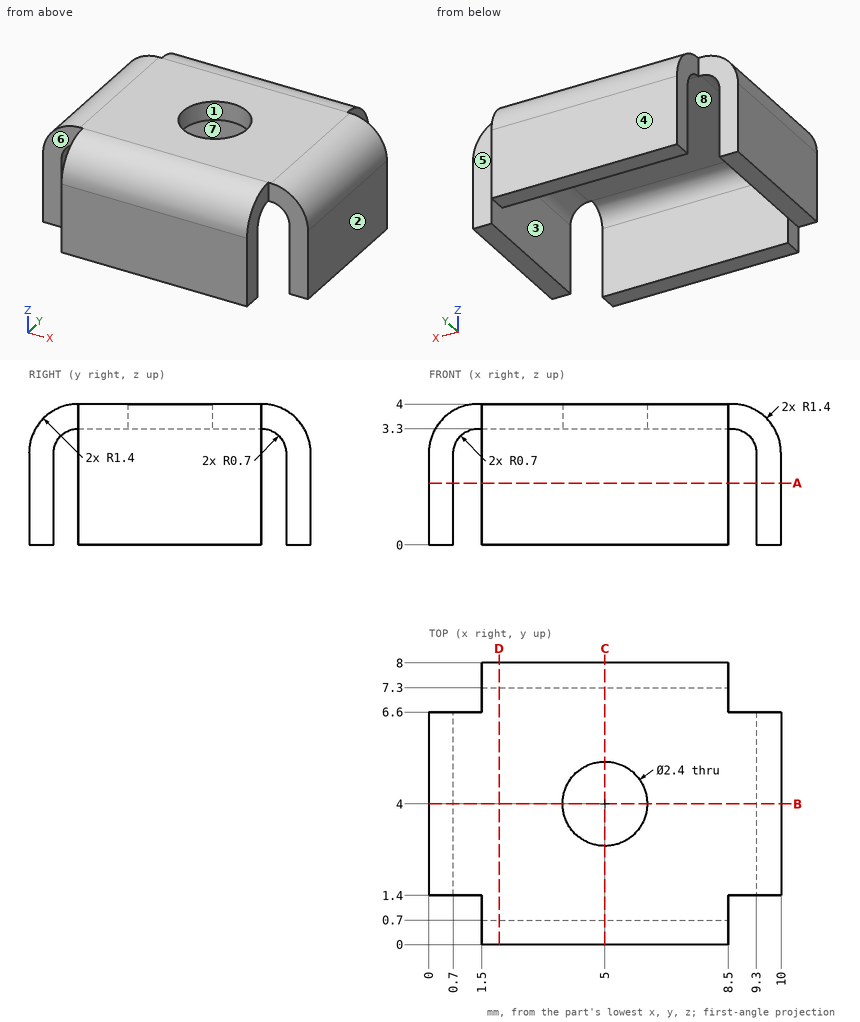
Geometry check sheet. Reference: drawing and pictorial views, mm from the part's lowest x, y, z. A direction names the side the tool comes from. Give positions to 0.01 mm unless a question says otherwise; leave off trailing zeros. Order: outer loops, then holes, each group sorted by start corner. A loop starts at its lowest first (then second) coordinate and runs counter-clockwise, first axis right, second up. Notation, with made-up numbers: (-2.5, 3) -> (2.5, 3) arc R25 cw to (2.5, 42) -> close; hole circle Ø11 at (87, 52). An arc over 180 degrees is marked (long way). Write each question's results on one line, items separated by ' | '. Start each with the question number.
(1) Mould release check, pull along X, two halves, no side actions. Record for the marked faces 1, 2, 3 and 4: pulls with the +X half, pulls with the -X half, needs draft (parallel to the pull), parting line crosses it, or undercut.
(2) Access from +Z, -Z, +X, -X, +Y, -Y to the whole of each face (thin tool, end or side, straight path). Record for the marked faces 5, 6, 7 and 8.
(3) Sectioned sample at A-A (z = 1.75). Enter the section's corners in (x, y).
(4) Gauge pin test, flat ends, axial feed: P1, Ø0.8, axis at x = 1, z = 2, coming from the -Y side; P2, Ø1.5, axis at y = 0.5, z = 2.5, coming from the -X side; P3, Ø0.5, axis at x = 0.5, z = 2, coming from the +Y side. Record the tip position at first contact, or that the pin passes through.
(5) Sectioned sample at C-C (x = 5). Enter the section's corners in (y, z), plus the area to 3 significant figures.
(6) Sectioned sample at B-B (y = 4). Enter the section's corners in (x, z), plus the area to 3 significant figures.
(7) Scan lines: line 1 (X direction, y = 2, z = 1); line 2 (Y direction, x = 7.25, z = 0.45); line 3 (Z direction, x = 3.75, y = 2.75). Record each from-to range of solid material in increasing order.
(8) Sectioned sample at D-D (x = 2). Enter the section's corners in (y, z), plus the area to 3 significant figures.
Answer below:
1) face 1: undercut | face 2: pulls with the +X half | face 3: undercut | face 4: needs draft
2) face 5: +Z, -Z, +X, +Y | face 6: +Z, -Z, -X, -Y | face 7: -Z, +X, -X | face 8: -Z
3) outline: (0, 1.4) -> (0.7, 1.4) -> (0.7, 6.6) -> (0, 6.6) -> close; (1.5, 0) -> (8.5, 0) -> (8.5, 0.7) -> (1.5, 0.7) -> close; (1.5, 7.3) -> (8.5, 7.3) -> (8.5, 8) -> (1.5, 8) -> close; (9.3, 1.4) -> (10, 1.4) -> (10, 6.6) -> (9.3, 6.6) -> close
4) P1: y = 1.4 | P2: x = 1.5 | P3: y = 6.6
5) outline: (0, 0) -> (0.7, 0) -> (0.7, 2.6) arc R0.7 cw to (1.4, 3.3) -> (2.8, 3.3) -> (2.8, 4) -> (1.4, 4) arc R1.4 ccw to (0, 2.6) -> close; (5.2, 3.3) -> (6.6, 3.3) arc R0.7 cw to (7.3, 2.6) -> (7.3, 0) -> (8, 0) -> (8, 2.6) arc R1.4 ccw to (6.6, 4) -> (5.2, 4) -> close | area: 7.91 mm2
6) outline: (0, 0) -> (0.7, 0) -> (0.7, 2.6) arc R0.7 cw to (1.4, 3.3) -> (3.8, 3.3) -> (3.8, 4) -> (1.4, 4) arc R1.4 ccw to (0, 2.6) -> close; (6.2, 3.3) -> (8.6, 3.3) arc R0.7 cw to (9.3, 2.6) -> (9.3, 0) -> (10, 0) -> (10, 2.6) arc R1.4 ccw to (8.6, 4) -> (6.2, 4) -> close | area: 9.31 mm2
7) line 1: 0 to 0.7, 9.3 to 10 | line 2: 0 to 0.7, 7.3 to 8 | line 3: 3.3 to 4
8) outline: (0, 0) -> (0.7, 0) -> (0.7, 2.6) arc R0.7 cw to (1.4, 3.3) -> (6.6, 3.3) arc R0.7 cw to (7.3, 2.6) -> (7.3, 0) -> (8, 0) -> (8, 2.6) arc R1.4 ccw to (6.6, 4) -> (1.4, 4) arc R1.4 ccw to (0, 2.6) -> close | area: 9.59 mm2
